from build123d import *

# Parameters (mm, degrees)
SKETCH1_W                 = 57.15
SKETCH1_H                 = 25.4
BOSS_EXTRUDE1_DEPTH       = 6.35
F_4_CLEARANCE_HOLE1_D     = 2.9464
F_4_CLEARANCE_HOLE1_DEPTH = 6.35
SKETCH4_R                 = 6.35
BOSS_EXTRUDE2_DEPTH       = 9.525
SKETCH5_R                 = 6.35
BOSS_EXTRUDE3_DEPTH       = 9.525
CUT_EXTRUDE1_DEPTH        = 5.08


with BuildPart() as part:
    # Sketch1 → Boss-Extrude1 (new body)
    with BuildSketch(Plane.XY):
        Rectangle(SKETCH1_W, SKETCH1_H)
    extrude(amount=BOSS_EXTRUDE1_DEPTH)

    # #4 Clearance Hole1
    with Locations(Plane.XY.offset(6.35)):
        with Locations((-22.225, 6.35), (22.225, -6.35), (-22.225, -6.35), (22.225, 6.35)):
            Hole(F_4_CLEARANCE_HOLE1_D / 2, depth=F_4_CLEARANCE_HOLE1_DEPTH)

    # Sketch4 → Boss-Extrude2 (add, symmetric)
    with BuildSketch(Plane(origin=(0, 0, 0), x_dir=(1, 0, 0), z_dir=(0, 1, 0))):
        with BuildLine():
            Line((-12.512025451, -40.276974762), (-18.415, -6.35))
            Line((-18.415, -6.35), (18.415, -6.35))
            Line((18.415, -6.35), (12.512025451, -40.276974762))
            ThreePointArc((12.512025451, -40.276974762), (0, -50.8), (-12.512025451, -40.276974762))
        make_face()
        with Locations((0, -38.1)):
            Circle(SKETCH4_R, mode=Mode.SUBTRACT)
    extrude(amount=BOSS_EXTRUDE2_DEPTH, both=True)

    # Sketch5 → Boss-Extrude3 (add, symmetric)
    with BuildSketch(Plane(origin=(0, 0, 0), x_dir=(1, 0, 0), z_dir=(0, 1, 0))):
        with BuildLine():
            Line((17.641611802, -10.795), (-17.641611802, -10.795))
            Line((-17.641611802, -10.795), (-12.512025451, -40.276974762))
            ThreePointArc((-12.512025451, -40.276974762), (0, -50.8), (12.512025451, -40.276974762))
            Line((12.512025451, -40.276974762), (17.641611802, -10.795))
        make_face()
        with Locations((0, -38.1)):
            Circle(SKETCH5_R, mode=Mode.SUBTRACT)
    extrude(amount=BOSS_EXTRUDE3_DEPTH, both=True)

    # Sketch6 → Cut-Extrude1 (cut, symmetric)
    with BuildSketch(Plane(origin=(0, 0, 0), x_dir=(1, 0, 0), z_dir=(0, 1, 0))):
        with BuildLine():
            Line((-16.691449159, -16.256), (16.691449159, -16.256))
            Line((16.691449159, -16.256), (12.512025451, -40.276974762))
            ThreePointArc((12.512025451, -40.276974762), (0, -50.8), (-12.512025451, -40.276974762))
            Line((-12.512025451, -40.276974762), (-16.691449159, -16.256))
        make_face()
    extrude(amount=CUT_EXTRUDE1_DEPTH, both=True, mode=Mode.SUBTRACT)


solid = part.part
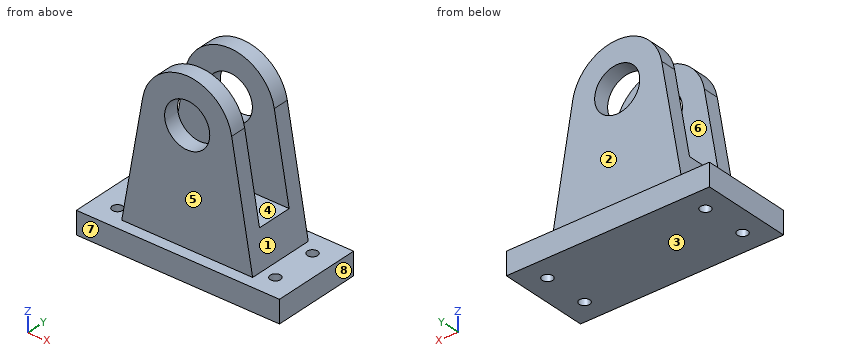
Part model, mm, in its own coordinate system. Face numbers are marked on the shaded views. A direction names the side the tool comes from. Give positions to 0.01 mm unless a question says otherwise; leave off trailing zeros. Write each loop counter-clockwise with the first axis right and the second up, starting at its lowest first coordinate (ties: lowest second). Pieces come first, ordered by that corner, then holes.
1) Cut at C-C on z = 38.1. Write the cut outline in (x, y) (3 decimals), then the cut area to 3 significant figures.
Resolved:
outline: (-12.891, -9.525) - (-6.35, -9.525) - (-6.35, -5.08) - (-12.891, -5.08) - close; (-12.891, 5.08) - (-6.35, 5.08) - (-6.35, 9.525) - (-12.891, 9.525) - close; (6.35, -9.525) - (12.891, -9.525) - (12.891, -5.08) - (6.35, -5.08) - close; (6.35, 5.08) - (12.891, 5.08) - (12.891, 9.525) - (6.35, 9.525) - close
area: 116 mm2
2) Pin check, flat tips, straight feed: pin 1 (3 mm diameter, centred on x = 0, y = -2, fed in from +Z); pin 2 (16.5 mm diameter, centred on x = -1, z = 41.5, fed in from +Y) (3 decimals); pin 3 (12 mm diameter, centred on x = 14.5, z = 25.5, fed in from -Y) (3 decimals). Stop position of each tip, or through.
Resolved:
pin 1: stops at z = 16.26
pin 2: stops at y = 9.525
pin 3: stops at y = -9.525
3) Which spindle directions (+Z, -Z, +X, -X, +Y, -Y) get a long thin tool onto all of the face, cutting with end or side? Do the marked faces 1, 2, 3, 4 and 5. Say none if no direction does.
Resolved:
face 1: +Z, +X, +Y, -Y
face 2: +Z, +X, -X, +Y
face 3: -Z, +X, -X, +Y, -Y
face 4: +Z, +X, -X
face 5: +Z, +X, -X, -Y
4) Two-plate mould, pull along Y, no slides. Class the marked faces 6, 7 and 8: released by +Y, released by -Y, zero draft, split by the parting line, or undercut.
Resolved:
face 6: undercut
face 7: released by -Y
face 8: zero draft
5) Probe L1, parallel to Z at x = 0, y = 6.2; L2, parallel to Y at x = -7.5, z = 34 (3 decimals); L3, parallel to Z at x = 26.5, y = -5.75. List the from-to ranges inside material, lowest first.
Resolved:
L1: z = 0 to 31.75, 44.45 to 50.8
L2: y = -9.525 to -5.08, 5.08 to 9.525
L3: z = 0 to 6.35
6) Cut at B-B on x = 0. Write the cut outline in (y, z) (3 decimals).
Resolved:
outline: (-12.7, 0) - (12.7, 0) - (12.7, 6.35) - (9.525, 6.35) - (9.525, 31.75) - (5.08, 31.75) - (5.08, 16.256) - (-5.08, 16.256) - (-5.08, 31.75) - (-9.525, 31.75) - (-9.525, 6.35) - (-12.7, 6.35) - close; (-9.525, 44.45) - (-5.08, 44.45) - (-5.08, 50.8) - (-9.525, 50.8) - close; (5.08, 44.45) - (9.525, 44.45) - (9.525, 50.8) - (5.08, 50.8) - close
7) Cut at A-A on y = -6.35. Write the cut outline in (x, z) (3 decimals), then the cut area to 3 significant figures.
Resolved:
outline: (-28.575, 0) - (-23.698, 0) - (-23.698, 6.35) - (-28.575, 6.35) - close; (-20.752, 0) - (20.752, 0) - (20.752, 6.35) - (18.415, 6.35) - (12.512, 40.277) arc R12.7 ccw to (-12.512, 40.277) - (-18.415, 6.35) - (-20.752, 6.35) - close; (23.698, 0) - (28.575, 0) - (28.575, 6.35) - (23.698, 6.35) - close; hole circle Ø12.7 at (0, 38.1)
area: 1,450 mm2
8) Cut at D-D on z = 22. Write the cut outline in (x, y) (3 decimals), then the cut area to 3 significant figures.
Resolved:
outline: (-15.692, -9.525) - (15.692, -9.525) - (15.692, -5.08) - (-15.692, -5.08) - close; (-15.692, 5.08) - (15.692, 5.08) - (15.692, 9.525) - (-15.692, 9.525) - close
area: 279 mm2
